The listing builds one solid part. Answer for the finished solid, in the listing's coordinates (mm). A direction names the side the tool comes from. Round coordinates to 2 decimals unless told otherwise and drop trailing zeros. Loops run counter-clockwise (first coordinate to the right, second up) from the corner with the lowest first, then second, coordinate; pieces in that order, holes last. Notation, with made-up numbers: M 43.5,-24 L 62.5,-24 A18 ccw 62.5,-13 Z; hole C 51,60.5 d9. An arc over 180 degrees is marked long. Put each result on its own line as item: value. Start each with the question number.
(1) Section B-B, the plane x = -14.25 is taken. Determine the outline of the cut face in (y, z).
(2) Which of the six approach directions +Z, -Z, +X, -X, +Y, -Y give full straight-line access (tool end or side, diameter ignored) to faces 1 (the face through (-14.8, -0.8, -10.4)), 2 (the face through (-19.768, -3.247, 8.329))?
(3) Section A-A, the plane z = 0 is taken. Determine the outline of the cut face in (x, y), then the cut area to 4 significant figures.
(4) Section D-D, the plane x = -20 is taken. Determine the outline of the cut face in (y, z).
(5) Determine the mould class of faces 3 (the face through (-19.768, 8.329, -3.247)), 4 (the face through (-15, 10, 0)), 5 (the face through (-15.93, 0.66, -14.985)), 6 (the face through (-21, -6, 6)) for opening direction Y: released by +Y, released by -Y, zero draft, split by the parting line, or undercut.
(6) Section C-C, the plane z = -3.25 is taken. Determine the outline of the cut face in (x, y).
(7) Flat-ended cylindrical pins translate along their axes: P1, Ø2, axis at x = -12.5, z = 9, coming from the +Y side; P2, Ø5, axis at x = -13.5, z = 3.5, coming from the -Y side; P3, Ø8, axis at y = -3, z = -2, coming from the -X side; P4, Ø2, axis at x = -13.5, y = -9.5, coming from the -Z side. Find the tip coordinate at first contact, or state that the pin passes through.
(8) Straight lines are drawn through the part: line 1 (Y direction, x = -13.5, z = 0); line 2 (Z direction, x = -19.5, y = -6.25); line 3 (X direction, y = -5.75, z = -0.25). For each, find the intervals that lie inside material, in ascending order.
```python
from build123d import *

# Parameters (mm, degrees)
SKETCH013_R             = 15
PAD008_DEPTH            = 10
POCKET002_DEPTH         = 2.5
POLARPATTERN_COUNT      = 4
SKETCH010_R             = 1
HOLE_DEPTH              = 25
POLARPATTERN001_COUNT   = 4
SKETCH011_R             = 4
POCKET001_DEPTH         = 7.501
BODY009_PLACEMENT_ANGLE = 90


with BuildPart() as part:
    # Sketch013 → Pad008 (new body)
    with BuildSketch(Plane.XY):
        Circle(SKETCH013_R)
    extrude(amount=PAD008_DEPTH)

    # Sketch012 (on Face3 of Pad008) → Pocket002 (cut)
    with BuildSketch(Plane.XY.offset(10)):
        with BuildLine():
            ThreePointArc((-5.26869, 1.578261), (0, -5.5), (5.26869, 1.578261))
            Line((2.107476, 12.131304), (5.26869, 1.578261))
            ThreePointArc((2.107476, 12.131304), (0, 13.7), (-2.107476, 12.131304))
            Line((-2.107476, 12.131304), (-5.26869, 1.578261))
        make_face()
    pocket002 = extrude(amount=-POCKET002_DEPTH, mode=Mode.SUBTRACT)

    # PolarPattern: Pocket002 ×4 about axis
    polarpattern_axis = Axis((0, 0, 10), (0, 0, 1))
    for i in range(1, POLARPATTERN_COUNT):
        add(pocket002.rotate(polarpattern_axis, i * 360 / POLARPATTERN_COUNT), mode=Mode.SUBTRACT)

    # Sketch010 (on Face21 of PolarPattern) → Hole (cut)
    with BuildSketch(Plane.XY.offset(7.5)):
        with Locations((0, 11)):
            Circle(SKETCH010_R)
    hole = extrude(amount=-HOLE_DEPTH, mode=Mode.SUBTRACT)

    # PolarPattern001: Hole ×4 about axis
    polarpattern001_axis = Axis((0, 0, 7.5), (0, 0, 1))
    for i in range(1, POLARPATTERN001_COUNT):
        add(hole.rotate(polarpattern001_axis, i * 360 / POLARPATTERN001_COUNT), mode=Mode.SUBTRACT)

    # Sketch011 (on Face25 of PolarPattern001) → Pocket001 (cut, through all)
    with BuildSketch(Plane.XY.offset(7.5)):
        Circle(SKETCH011_R)
    extrude(amount=-POCKET001_DEPTH, mode=Mode.SUBTRACT)


with BuildPart() as part_1:
    # Body009 placement: moved
    add(part.part.moved(Location((-11, 0, 0))).rotate(Axis((-11, 0, 0), (0, -1, 0)), BODY009_PLACEMENT_ANGLE))


solid = part_1.part
```
Recorded:
1. outline: C 0,0 d30; hole C -11,0 d2; hole C 0,0 d8; hole C 0,-11 d2; hole C 0,11 d2; hole C 11,0 d2
2. face 1: +X, -X
2. face 2: -X
3. outline: M -21,-15 L -11,-15 L -11,-12 L -18.5,-12 L -18.5,-13.7 L -21,-13.7 Z; M -21,13.7 L -18.5,13.7 L -18.5,12 L -11,12 L -11,15 L -21,15 Z; M -18.5,-10 L -11,-10 L -11,-4 L -18.5,-4 Z; M -18.5,4 L -11,4 L -11,10 L -18.5,10 Z
3. area: 141.5 mm²
4. outline: C 0,0 d30; hole M -12.13,-2.11 L -4.42,-4.42 L -2.11,-12.13 A2.2 ccw 2.11,-12.13 L 4.42,-4.42 L 12.13,-2.11 A2.2 ccw 12.13,2.11 L 4.42,4.42 L 2.11,12.13 A2.2 ccw -2.11,12.13 L -4.42,4.42 L -12.13,2.11 A2.2 ccw Z
5. face 3: undercut
5. face 4: undercut
5. face 5: split by the parting line
5. face 6: zero draft
6. outline: M -21,-14.64 L -11,-14.64 L -11,-2.33 L -18.5,-2.33 L -18.5,-8.32 L -21,-8.32 Z; M -21,8.32 L -18.5,8.32 L -18.5,2.33 L -11,2.33 L -11,14.64 L -21,14.64 Z
7. P1: stops at y = 12.69
7. P2: stops at y = -14.97
7. P3: stops at x = -21
7. P4: stops at z = -12.36
8. line 1: y = -15 to -12, -10 to -4, 4 to 10, 12 to 15
8. line 2: z = -13.64 to -3.87, 3.87 to 13.64
8. line 3: x = -18.5 to -11
